Job drawing, mm, ordinate dimensions from the low corner. One solid piece. Coordinates: 2 decimals unless noted, no trailing zeros. Loops run counter-clockwise (first coordinate to the right, second up) from the corner with the lowest first, then second, coordinate; pieces in that order, holes last. Notation, with made-up numbers: (48, -40) - (73, -40) arc R12 cw to (73, -22) - close; hole circle Ø6 at (1.5, 17.5). An arc over 180 degrees is marked (long way). Use a Markdown table: item, result. Add a question column.
1. Drop a flat-ended pin along its axis: pin 1 (22.5 mm diameter, centred on x = 75, z = 75, fed in from +Y). Give the stop position or say it passes through.
2. Wall check: probe 1 along X at (y, z) = (28.5, 75). Give the ranges that are in metal, low to high. Write a range as [from, to].
3. Band-saw the part on B-B, the plane z = 675. Give the cut face in (x, y).
4. Band-saw the part on A-A, the plane x = 675. Give the cut face in (y, z), plus the area to 3 significant figures.
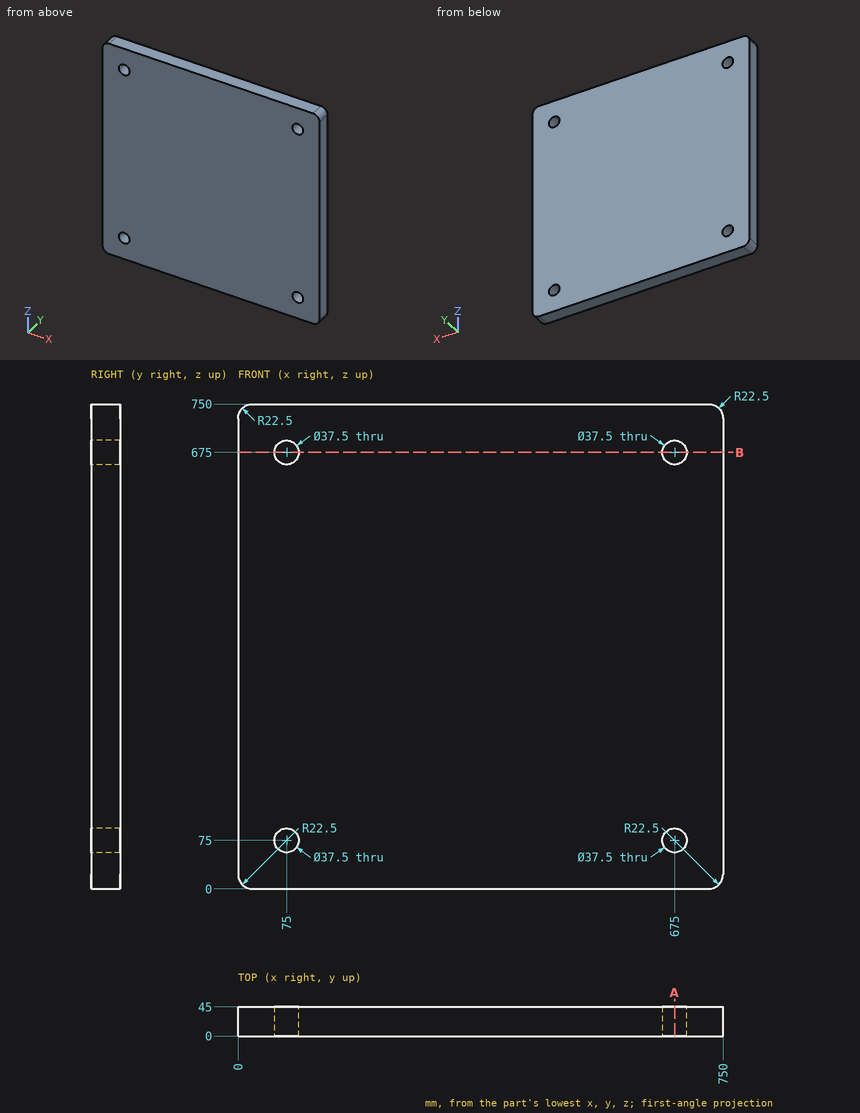
Geometry check:
| question | item | result |
|---|---|---|
| 1 | pin 1 | passes through |
| 2 | probe 1 | x = [0, 56.25], [93.75, 656.25], [693.75, 750] |
| 3 | outline | (0, 0) - (56.25, 0) - (56.25, 45) - (0, 45) - close; (93.75, 0) - (656.25, 0) - (656.25, 45) - (93.75, 45) - close; (693.75, 0) - (750, 0) - (750, 45) - (693.75, 45) - close |
| 4 | outline | (0, 0) - (45, 0) - (45, 56.25) - (0, 56.25) - close; (0, 93.75) - (45, 93.75) - (45, 656.25) - (0, 656.25) - close; (0, 693.75) - (45, 693.75) - (45, 750) - (0, 750) - close |
| 4 | area | 30,400 mm^2 |
